Verification items for the finished model (mm, model axes). A direction names the side the tool comes from. Give positions to 0.01 mm unless a question says otherwise; leave off trailing zeros. Order: outer loops, then holes, each group sorted by start corner. A loop starts at its lowest first (then second) coordinate and runs counter-clockwise, first axis right, second up. Notation, with made-up numbers: (-14, -20) -> (35, -20) arc R16 ccw to (35, -12) -> close; hole circle Ø2 at (46, 47.25). An arc over 180 degrees is marked (long way). Return JSON: item names as keys, results as strings. Group by question number.
(1) Cross-section at B-B on x = -5. Enter the section's corners in (y, z).
(2) Depth check by flat-ended pin: pin 1 Ø3.5 at (x, z) = (-46.46, 0) entering from +Y; pin 2 Ø6 at (y, z) = (-19.5, 37) entering from +X; pin 3 Ø10 at (y, z) = (-6.5, 14) entering from +X. Enter the tip coordinate at first touch or a pass-through.
(3) Cross-section at A-A on y = -2.5. Enter the section's corners in (x, z), then the cut area to 3 significant figures.
(4) Tool access check on faces 5 (the face through (78.043, -18.783, 21.51)), 6 (the face through (-5, -19, 18.959)), 7 (the face through (50.61, -18.78, 37.64)), 8 (the face through (78.903, -19, 6)). Record the directions out of +Z, -Z, +X, -X, +Y, -Y that give a thin tool (end or side, any length) a straight path to the whole face; none if there is none.
(5) Thickness scan on line 1 along Z through (x, y) = (11.5, -9.5); line 2 along X through (y, z) = (-14, -2.5); line 3 along X through (y, z) = (-25, 13.5). Record the ranges inside material, lowest first.
(6) Cross-section at C-C on z = 0. Enter the section's corners in (x, y), then the cut area to 3 significant figures.
(7) Cross-section at D-D on x = 39.5. Enter the section's corners in (y, z).
(8) Release check for a two-part mould opening along Z. For faces 1 (the face through (-1, -19, -6.35)), 2 (the face through (-1, 0, 15)), 3 (the face through (77.79, -18.78, 27.84)), 4 (the face through (54.84, -19, 26)) record: pulls with the +Z half, pulls with the -Z half, needs draft (parallel to the pull), parting line crosses it, or undercut.
from build123d import *

# Parameters (mm, degrees)
F0_R     = 3
F1_DEPTH = 38.1


with BuildPart() as f1:
    # F0 (on Front) → F1 (new body)
    with BuildSketch(Plane.XZ):
        with BuildLine():
            ThreePointArc((-63.834237, -6.35), (-49.682526, 18.216848), (-27.958176, 0))
            ThreePointArc((-27.958176, 0), (-28.241328, -3.22435), (-29.082115, -6.35))
            Line((-29.082115, -6.35), (29.656009, -6.35))
            ThreePointArc((29.656009, -6.35), (43.80772, 18.216848), (65.53207, 0))
            ThreePointArc((65.53207, 0), (65.248919, -3.22435), (64.408131, -6.35))
            Line((64.408131, -6.35), (78.902803, -6.35))
            Line((78.902803, -6.35), (78.902803, 18.319092))
            ThreePointArc((78.902803, 18.319092), (78.019117, 21.550487), (75.614012, 23.8825))
            Line((75.614012, 23.8825), (80.032745, 31.913057))
            Line((80.032745, 31.913057), (77.126751, 33.512051))
            Line((77.126751, 33.512051), (68.966064, 27.540465))
            Line((68.966064, 27.540465), (31.739181, 48.02418))
            ThreePointArc((31.739181, 48.02418), (30.258299, 48.610981), (28.677972, 48.810773))
            Line((28.677972, 48.810773), (-21.916144, 48.810773))
            Line((-21.916144, 48.810773), (-29.875312, 29.312046))
            Line((-29.875312, 29.312046), (-73.56282, 22.273607))
            ThreePointArc((-73.56282, 22.273607), (-77.386855, 20.122025), (-78.902803, 16.004447))
            Line((-78.902803, 16.004447), (-78.902803, -6.35))
            Line((-78.902803, -6.35), (-63.834237, -6.35))
        make_face()
        Polygon((-27.242659, 18.959029), (-17.649503, 42.460773), (22.330722, 42.460773), (17.231188, 18.959029), align=None, mode=Mode.SUBTRACT)
        Polygon((23.578439, 18.959029), (28.677972, 42.460773), (54.840085, 28.065335), (54.840085, 23.482008), align=None, mode=Mode.SUBTRACT)
        with BuildLine():
            ThreePointArc((-29.082115, -6.35), (-28.241328, -3.22435), (-27.958176, 0))
            ThreePointArc((-27.958176, 0), (-49.682526, 18.216848), (-63.834237, -6.35))
            Line((-63.834237, -6.35), (-29.082115, -6.35))
        make_face()
        with Locations((-46.458176, 0)):
            Circle(F0_R, mode=Mode.SUBTRACT)
        with BuildLine():
            ThreePointArc((65.53207, 0), (43.80772, 18.216848), (29.656009, -6.35))
            Line((29.656009, -6.35), (64.408131, -6.35))
            ThreePointArc((64.408131, -6.35), (65.248919, -3.22435), (65.53207, 0))
        make_face()
        with Locations((47.03207, 0)):
            Circle(F0_R, mode=Mode.SUBTRACT)
    extrude(amount=F1_DEPTH)


solid = f1.part
Verdict:
{
 "1": {"outline": "(-38.1, -6.35) -> (0, -6.35) -> (0, 18.96) -> (-38.1, 18.96) -> close; (-38.1, 42.46) -> (0, 42.46) -> (0, 48.81) -> (-38.1, 48.81) -> close"},
 "2": {"pin 1": "through", "pin 2": "x = 57.23", "pin 3": "x = 78.9"},
 "3": {"outline": "(-78.9, -6.35) -> (78.9, -6.35) -> (78.9, 18.32) arc R6.35 ccw to (75.61, 23.88) -> (80.03, 31.91) -> (77.13, 33.51) -> (68.97, 27.54) -> (31.74, 48.02) arc R6.35 ccw to (28.68, 48.81) -> (-21.92, 48.81) -> (-29.88, 29.31) -> (-73.56, 22.27) arc R6.35 ccw to (-78.9, 16) -> close; hole circle Ø6 at (-46.46, 0); hole (-27.24, 18.96) -> (17.23, 18.96) -> (22.33, 42.46) -> (-17.65, 42.46) -> close; hole (23.58, 18.96) -> (54.84, 23.48) -> (54.84, 28.07) -> (28.68, 42.46) -> close; hole circle Ø6 at (47.03, 0)", "area": "5,400 mm²"},
 "4": {"face 5": "+X, +Y, -Y", "face 6": "+Y, -Y", "face 7": "+Z, +Y, -Y", "face 8": "-Z, +X, +Y, -Y"},
 "5": {"line 1": "-6.35 to 18.96, 42.46 to 48.81", "line 2": "-78.9 to -48.12, -44.8 to 45.37, 48.69 to 78.9", "line 3": "-78.9 to 78.9"},
 "6": {"outline": "(-78.9, -38.1) -> (-49.46, -38.1) -> (-49.46, 0) -> (-78.9, 0) -> close; (-43.46, -38.1) -> (44.03, -38.1) -> (44.03, 0) -> (-43.46, 0) -> close; (50.03, -38.1) -> (78.9, -38.1) -> (78.9, 0) -> (50.03, 0) -> close", "area": "5,560 mm²"},
 "7": {"outline": "(-38.1, -6.35) -> (0, -6.35) -> (0, 21.26) -> (-38.1, 21.26) -> close; (-38.1, 36.51) -> (0, 36.51) -> (0, 43.75) -> (-38.1, 43.75) -> close"},
 "8": {"face 1": "pulls with the -Z half", "face 2": "needs draft", "face 3": "undercut", "face 4": "undercut"}
}
